```python
from build123d import *

# Parameters (mm, degrees)
BOSS_EXTRUDE2_DEPTH = 1.5875


with BuildPart() as part:
    # Sketch2 → Boss-Extrude2 (new body)
    with BuildSketch(Plane.XY):
        with BuildLine():
            Line((0, 0), (22.726605384, 0))
            Line((22.726605384, 0), (25.4, 0))
            Line((25.4, 0), (93.218, 0))
            Line((93.218, 0), (93.218, 25.4))
            Line((93.218, 25.4), (76.2, 266.7))
            Line((76.2, 266.7), (57.898403378, 266.7))
            Line((57.898403378, 266.7), (58.118386132, 263.580841559))
            ThreePointArc((58.118386132, 263.580841559), (57.382444397, 262.733216707), (56.534819546, 263.469158441))
            Line((56.534819546, 263.469158441), (56.306960194, 266.7))
            Line((56.306960194, 266.7), (25.4, 266.7))
            Line((25.4, 266.7), (25.4, 26.9875))
            ThreePointArc((25.4, 26.9875), (24.935032015, 25.864967985), (23.8125, 25.4))
            Line((23.8125, 25.4), (0, 25.4))
            Line((0, 25.4), (0, 0))
        make_face()
        with BuildLine():
            Line((34.777339087, 260.35), (68.802586709, 260.35))
            ThreePointArc((68.802586709, 260.35), (69.884912746, 259.92384689), (70.386153295, 258.874183117))
            Line((70.386153295, 258.874183117), (74.25178186, 204.063031823))
            ThreePointArc((74.25178186, 204.063031823), (73.194086522, 202.453478324), (71.362368826, 203.048618789))
            Line((71.362368826, 203.048618789), (61.367737995, 217.506379541))
            Line((61.367737995, 217.506379541), (61.713239359, 212.607479611))
            ThreePointArc((61.713239359, 212.607479611), (60.966778576, 211.777785767), (60.128358495, 212.514431775))
            Line((60.128358495, 212.514431775), (59.595490006, 220.070029749))
            Line((59.595490006, 220.070029749), (33.471492639, 257.859770083))
            ThreePointArc((33.471492639, 257.859770083), (33.371415904, 259.499749112), (34.777339087, 260.35))
        make_face(mode=Mode.SUBTRACT)
        with BuildLine():
            Line((81.657258841, 99.06), (85.652951472, 42.404656719))
            ThreePointArc((85.652951472, 42.404656719), (84.6981432, 40.835297632), (82.901413184, 41.217799964))
            Line((82.901413184, 41.217799964), (73.045756556, 51.924096733))
            Line((73.045756556, 51.924096733), (73.333849522, 47.839196468))
            ThreePointArc((73.333849522, 47.839196468), (72.597907788, 46.991571616), (71.750282937, 47.727513351))
            Line((71.750282937, 47.727513351), (71.322271249, 53.796335779))
            Line((71.322271249, 53.796335779), (32.106028298, 96.397326362))
            ThreePointArc((32.106028298, 96.397326362), (31.820212808, 98.110198243), (33.274, 99.06))
            Line((33.274, 99.06), (81.657258841, 99.06))
        make_face(mode=Mode.SUBTRACT)
        with BuildLine():
            Line((31.75, 26.9875), (31.75, 83.339802581))
            ThreePointArc((31.75, 83.339802581), (32.76043797, 84.818706115), (34.505471702, 84.414976219))
            Line((34.505471702, 84.414976219), (86.380452981, 28.062673638))
            ThreePointArc((86.380452981, 28.062673638), (86.666268471, 26.349801757), (85.212481279, 25.4))
            Line((85.212481279, 25.4), (74.916403378, 25.4))
            Line((74.916403378, 25.4), (75.136386132, 22.280841559))
            ThreePointArc((75.136386132, 22.280841559), (74.400444397, 21.433216707), (73.552819546, 22.169158441))
            Line((73.552819546, 22.169158441), (73.324960194, 25.4))
            Line((73.324960194, 25.4), (33.3375, 25.4))
            ThreePointArc((33.3375, 25.4), (32.214967985, 25.864967985), (31.75, 26.9875))
        make_face(mode=Mode.SUBTRACT)
        with BuildLine():
            Line((79.221902862, 107.970834504), (34.591603741, 165.475243131))
            ThreePointArc((34.591603741, 165.475243131), (32.823074805, 166.003748488), (31.75, 164.501908627))
            Line((31.75, 164.501908627), (31.75, 106.9975))
            ThreePointArc((31.75, 106.9975), (32.214967985, 105.874967985), (33.3375, 105.41))
            Line((33.3375, 105.41), (67.682149668, 105.41))
            Line((67.682149668, 105.41), (67.91000902, 102.179158441))
            ThreePointArc((67.91000902, 102.179158441), (68.757633871, 101.443216707), (69.493575605, 102.290841559))
            Line((69.493575605, 102.290841559), (69.273592852, 105.41))
            Line((69.273592852, 105.41), (77.967799122, 105.41))
            ThreePointArc((77.967799122, 105.41), (79.393513815, 106.299292393), (79.221902862, 107.970834504))
        make_face(mode=Mode.SUBTRACT)
        with BuildLine():
            Line((34.991617614, 179.493333333), (74.505109516, 179.493333333))
            ThreePointArc((74.505109516, 179.493333333), (75.587435553, 179.067180223), (76.088676102, 178.01751645))
            Line((76.088676102, 178.01751645), (80.038176523, 122.017137338))
            ThreePointArc((80.038176523, 122.017137338), (79.021577531, 120.42265147), (77.200506197, 120.932119716))
            Line((77.200506197, 120.932119716), (67.277133916, 133.717999844))
            Line((67.277133916, 133.717999844), (67.59537819, 129.205581031))
            ThreePointArc((67.59537819, 129.205581031), (66.859436456, 128.357956179), (66.011811604, 129.093897913))
            Line((66.011811604, 129.093897913), (65.526620874, 135.973467973))
            Line((65.526620874, 135.973467973), (33.737513874, 176.932498829))
            ThreePointArc((33.737513874, 176.932498829), (33.56590292, 178.60404094), (34.991617614, 179.493333333))
        make_face(mode=Mode.SUBTRACT)
        with BuildLine():
            Line((73.81525743, 188.333563251), (34.643346448, 244.997798955))
            ThreePointArc((34.643346448, 244.997798955), (32.86467603, 245.610520701), (31.75, 244.095069038))
            Line((31.75, 244.095069038), (31.75, 187.430833333))
            ThreePointArc((31.75, 187.430833333), (32.214967985, 186.308301318), (33.3375, 185.843333333))
            Line((33.3375, 185.843333333), (62.009483001, 185.843333333))
            Line((62.009483001, 185.843333333), (62.237342353, 182.612491775))
            ThreePointArc((62.237342353, 182.612491775), (63.084967204, 181.87655004), (63.820908939, 182.724174892))
            Line((63.820908939, 182.724174892), (63.600926185, 185.843333333))
            Line((63.600926185, 185.843333333), (72.509410982, 185.843333333))
            ThreePointArc((72.509410982, 185.843333333), (73.915334165, 186.693584221), (73.81525743, 188.333563251))
        make_face(mode=Mode.SUBTRACT)
    extrude(amount=BOSS_EXTRUDE2_DEPTH)


solid = part.part
```
Geometry: final body of the model. Coordinates: model frame, mm. A direction names the side the tool comes from. Coordinates: 2 decimals unless noted, no trailing zeros. Write each loop counter-clockwise with the first axis right and the second up, starting at its lowest first coordinate (ties: lowest second). Pieces come first, ordered by that corner, then holes. Notation, with made-up numbers: M 42.5,70 L 68.5,70 A21 ccw 68.5,90 Z; hole C 73.25,-13.75 d6. An arc over 180 degrees is marked long. Answer as CSV lines item,"result". Start each with the question number.
Q1. Line query: line 1 (X direction, y = 212.5, z = 0.85); line 2 (X direction, y = 149, z = 0.4); line 3 (X direction, y = 151.5, z = 0.75). Output: solid intervals per line, ascending. Write a range as from..to.
Q2. Reachability of faces 4 (the flat face through (50, 104, 0)), 5 (the flat face through (57.22, 136.32, 0.78)) from +Z, -Z, +X, -X, +Y, -Y: full face, straight path, thin tool, end or side. Return the list, or none.
Q3. Cut plane B-B on y = 79.5. Return the cut outline in (x, z).
Q4. Cut plane C-C on y = 112.5. Return the cut outline in (x, z).
Q5. Pin query (flat end, axial travel): P1, Ø0.8, axis at x = 7.5, z = 1, coming from the +Y side; P2, Ø0.5, axis at y = 209.5, z = 0.5, coming from the +X side; P3, Ø0.5, axis at y = 54.5, z = 1, coming from the +X side. Return the tip coordinate at first contact, or that it passes through.
Q6. Mould query, pull axis Y, two halves, no side actions, for faces 1 (the flat face through (78.04, 46.5, 0.78)), 2 (the flat face through (50, 104, 1.588)), 3 (the flat face through (84.83, 144.36, 0.78)). Classes: released by +Y, released by -Y, zero draft, split by the parting line, or undercut.
Q7. Cut plane D-D on z = 1.1. Count the separate pieces of the cut face and the enclosed holes in it, then the cut area to 3 significant figures.
Q8. Cut plane A-A on x = 40. Return the cut outline in (y, z).
Findings below:
1,line 1,"x = 25.4..31.75, 57.11..60.13, 61.71..64.83, 73.66..80.02"
1,line 2,"x = 25.4..31.75, 47.38..55.42, 78.14..84.5"
1,line 3,"x = 25.4..31.75, 45.44..53.48, 77.96..84.32"
2,face 4,"-Z, +X, -X, +Y, -Y"
2,face 5,"+Z, -Z"
3,outline,"M 25.4,0 L 31.75,0 L 31.75,1.59 L 25.4,1.59 Z; M 39.03,0 L 47.66,0 L 47.66,1.59 L 39.03,1.59 Z; M 83.04,0 L 89.4,0 L 89.4,1.59 L 83.04,1.59 Z"
4,outline,"M 25.4,0 L 31.75,0 L 31.75,1.59 L 25.4,1.59 Z; M 75.71,0 L 87.08,0 L 87.08,1.59 L 75.71,1.59 Z"
5,P1,"stops at y = 25.4"
5,P2,"stops at x = 80.25"
5,P3,"stops at x = 91.18"
6,face 1,"undercut"
6,face 2,"zero draft"
6,face 3,"released by +Y"
7,separate pieces,"1"
7,enclosed holes,"6"
7,area,"7,760 mm2"
8,outline,"M 0,0 L 25.4,0 L 25.4,1.59 L 0,1.59 Z; M 78.45,0 L 87.82,0 L 87.82,1.59 L 78.45,1.59 Z; M 99.06,0 L 105.41,0 L 105.41,1.59 L 99.06,1.59 Z; M 158.51,0 L 168.86,0 L 168.86,1.59 L 158.51,1.59 Z; M 179.49,0 L 185.84,0 L 185.84,1.59 L 179.49,1.59 Z; M 237.25,0 L 248.42,0 L 248.42,1.59 L 237.25,1.59 Z; M 260.35,0 L 266.7,0 L 266.7,1.59 L 260.35,1.59 Z"
